Could you check a few things on this drawing? It's one solid part, dimensions in mm from its lowest x, y, z. Coordinates: 2 decimals unless noted, no trailing zeros. Write each loop counter-clockwise with the first axis right and the second up, starting at its lowest first coordinate (ties: lowest second). Pieces come first, ordered by that corner, then holes. Notation, with made-up numbers: (60, 30.25) - (80, 30.25) arc R20 cw to (80, 47.25) - close; hole circle Ø1 at (88, 53.25). An arc over 180 degrees is marked (long way). Answer as a JSON object with one key per item and string values. Group by question number.
1) If we section it at B-B (z = 250): Write out the boundary of the cut face in (x, y).
2) If we section it at D-D (x = 425.5): Write out the boundary of the cut face in (y, z).
3) If we section it at A-A (y = 16): Write out the boundary of the cut face in (x, z), plus the area to 3 significant figures.
4) Please list where these lines run through material, in increasing order: line 1 along X through (y, z) = (14, 250); line 2 along Z through (x, y) = (324, 18.25); line 3 along X through (y, z) = (5, 250).
5) Will these pins go through, and if not, where does the flat tip stop? pin 1 Ø10 at (y, z) = (14.5, 407.5) entering from -X; pin 2 Ø10 at (x, y) = (344.5, 12.5) entering from +Z; pin 3 Ø2 at (y, z) = (10.5, 121.5) entering from -X.
6) If we section it at C-C (x = 250): Write out the boundary of the cut face in (y, z), plus the area to 4 significant figures.
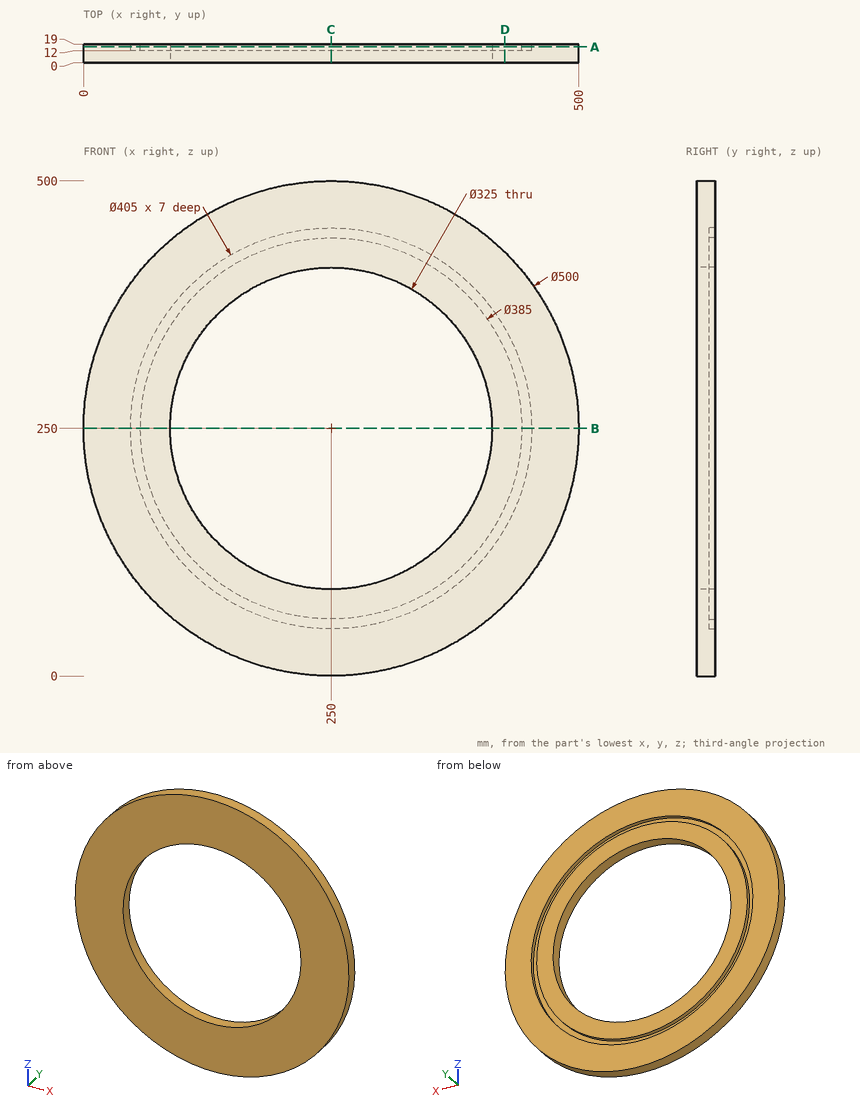
Here are the results:
{
 "1": {"outline": "(0, 0) - (87.5, 0) - (87.5, 19) - (57.5, 19) - (57.5, 12) - (47.5, 12) - (47.5, 19) - (0, 19) - close; (412.5, 0) - (500, 0) - (500, 19) - (452.5, 19) - (452.5, 12) - (442.5, 12) - (442.5, 19) - (412.5, 19) - close"},
 "2": {"outline": "(0, 71.96) - (19, 71.96) - (19, 148.98) - (12, 148.98) - (12, 170.91) - (19, 170.91) - (19, 329.09) - (12, 329.09) - (12, 351.02) - (19, 351.02) - (19, 428.04) - (0, 428.04) - close"},
 "3": {"outline": "circle Ø500 at (250, 250); circle Ø385 at (250, 250); hole circle Ø405 at (250, 250); hole circle Ø325 at (250, 250)", "area": "101,000 mm²"},
 "4": {"line 1": "x = 0 to 47.5, 57.5 to 87.5, 412.5 to 442.5, 452.5 to 500", "line 2": "z = 11.2 to 61.51, 72.29 to 105.33, 394.67 to 427.71, 438.49 to 488.8", "line 3": "x = 0 to 87.5, 412.5 to 500"},
 "5": {"pin 1": "stops at x = 51.9", "pin 2": "stops at z = 483.43", "pin 3": "stops at x = 34.96"},
 "6": {"outline": "(0, 0) - (19, 0) - (19, 47.5) - (12, 47.5) - (12, 57.5) - (19, 57.5) - (19, 87.5) - (0, 87.5) - close; (0, 412.5) - (19, 412.5) - (19, 442.5) - (12, 442.5) - (12, 452.5) - (19, 452.5) - (19, 500) - (0, 500) - close", "area": "3,185 mm²"}
}
